Here's how the part is built. I have some questions about the finished solid (model axes, mm). Round coordinates to 2 decimals unless told otherwise and drop trailing zeros. Answer as a JSON object with one key per item and string values.
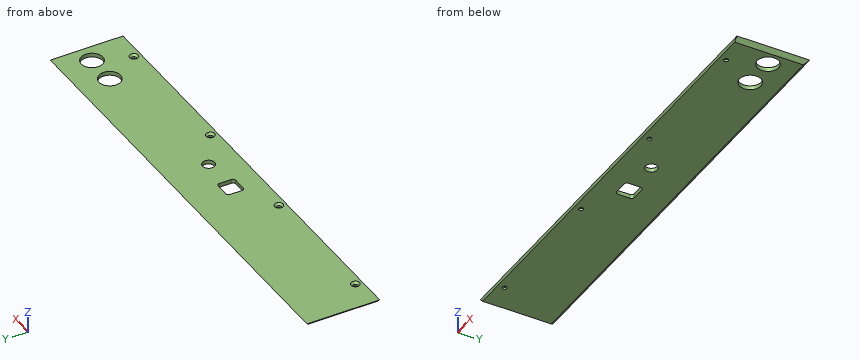
from build123d import *

# Parameters (mm, degrees)
SKETCH1_W                                      = 335.5
SKETCH1_H                                      = 54
BOSS_EXTRUDE1_DEPTH                            = 3
CHAMFER1_SIZE                                  = 3
CSK_FOR_M3_FLAT_HEAD_MACHINE_SCREW1_AT_2_COUNT = 2
CSK_FOR_M3_FLAT_HEAD_MACHINE_SCREW1_AT_2_PITCH = 100
CSK_FOR_M3_FLAT_HEAD_MACHINE_SCREW1_AT_3_COUNT = 2
CSK_FOR_M3_FLAT_HEAD_MACHINE_SCREW1_AT_3_PITCH = 189.5
CSK_FOR_M3_FLAT_HEAD_MACHINE_SCREW1_AT_4_COUNT = 2
CSK_FOR_M3_FLAT_HEAD_MACHINE_SCREW1_AT_4_PITCH = 289.5
SKETCH5_R                                      = 4.5
SKETCH5_R_2                                    = 8
CUT_EXTRUDE1_DEPTH                             = 340.831208102


with BuildPart() as part:
    # Sketch1 → Boss-Extrude1 (new body)
    with BuildSketch(Plane.XY):
        with Locations((167.75, 27)):
            Rectangle(SKETCH1_W, SKETCH1_H)
    extrude(amount=BOSS_EXTRUDE1_DEPTH)

    # Chamfer1
    chamfer1_edges = [part.edges().sort_by_distance(p)[0] for p in [
        (0, 27, 0),
        (167.75, 54, 0),
        (335.5, 27, 0),
    ]]
    chamfer(chamfer1_edges, length=CHAMFER1_SIZE - 0.0001)  # a hair under: the kernel refuses the full size

    # Sketch3 → CSK for M3 Flat Head Machine Screw1 (revolve, cut)
    with BuildSketch(Plane(origin=(23, 5, 3), x_dir=(0, -1, 0), z_dir=(1, 0, 0))):
        Polygon((0, 0), (0, 3), (1.7, 3), (1.7, 1.45), (3.15, 0), align=None)
    csk_for_m3_flat_head_machine_screw1 = revolve(axis=Axis((23, 5, 9.35), (0, 0, -1)), mode=Mode.SUBTRACT)

    # CSK for M3 Flat Head Machine Screw1 at 2: CSK for M3 Flat Head Machine Screw1 ×2
    with Locations(*[(i * CSK_FOR_M3_FLAT_HEAD_MACHINE_SCREW1_AT_2_PITCH, 0, 0) for i in range(1, CSK_FOR_M3_FLAT_HEAD_MACHINE_SCREW1_AT_2_COUNT)]):
        add(csk_for_m3_flat_head_machine_screw1, mode=Mode.SUBTRACT)

    # CSK for M3 Flat Head Machine Screw1 at 3: CSK for M3 Flat Head Machine Screw1 ×2
    with Locations(*[(i * CSK_FOR_M3_FLAT_HEAD_MACHINE_SCREW1_AT_3_PITCH, 0, 0) for i in range(1, CSK_FOR_M3_FLAT_HEAD_MACHINE_SCREW1_AT_3_COUNT)]):
        add(csk_for_m3_flat_head_machine_screw1, mode=Mode.SUBTRACT)

    # CSK for M3 Flat Head Machine Screw1 at 4: CSK for M3 Flat Head Machine Screw1 ×2
    with Locations(*[(i * CSK_FOR_M3_FLAT_HEAD_MACHINE_SCREW1_AT_4_PITCH, 0, 0) for i in range(1, CSK_FOR_M3_FLAT_HEAD_MACHINE_SCREW1_AT_4_COUNT)]):
        add(csk_for_m3_flat_head_machine_screw1, mode=Mode.SUBTRACT)

    # Sketch5 → Cut-Extrude1 (cut, through all)
    with BuildSketch(Plane.XY.offset(3)):
        with Locations((184.9, 22)):
            Circle(SKETCH5_R)
        with Locations((298.7, 30.75)):
            Circle(SKETCH5_R_2)
        with Locations((321.9, 30.75)):
            Circle(SKETCH5_R_2)
        with BuildLine():
            Line((151, 28.5), (161, 28.5))
            ThreePointArc((161, 28.5), (162.414213562, 27.914213562), (163, 26.5))
            Line((163, 26.5), (163, 17.5))
            ThreePointArc((163, 17.5), (162.414213562, 16.085786438), (161, 15.5))
            Line((161, 15.5), (151, 15.5))
            ThreePointArc((151, 15.5), (149.585786438, 16.085786438), (149, 17.5))
            Line((149, 17.5), (149, 26.5))
            ThreePointArc((149, 26.5), (149.585786438, 27.914213562), (151, 28.5))
        make_face()
    extrude(amount=-CUT_EXTRUDE1_DEPTH, mode=Mode.SUBTRACT)


solid = part.part
Item 1: Please list where these lines run through material, in increasing order: probe 1 along X at (y, z) = (6.5, 1.95); probe 2 along X at (y, z) = (18.5, 1.8); probe 3 along X at (y, z) = (5, 1.1). Write a range as from..to.
Resolved:
{"probe 1": "1.05..21.53, 24.47..121.53, 124.47..211.03, 213.97..311.03, 313.97..334.45", "probe 2": "1.2..149, 163..182.07, 187.73..334.3", "probe 3": "1.9..21.3, 24.7..121.3, 124.7..210.8, 214.2..310.8, 314.2..333.6"}
Item 2: I want a section at B-B, the plane y = 35. State how many separate pieces and enclosed holes the cut face has, then the cut area to 3 significant figures.
Resolved:
{"separate pieces": "3", "enclosed holes": "0", "area": "916 mm²"}
Item 3: I'm going to push flat-ended pins straight in: pin 1 Ø1.5 at (y, z) = (23, 2) entering from -X; pin 2 Ø0.9 at (y, z) = (22, 1) entering from +X; pin 3 Ø1.5 at (x, z) = (157.5, 1.5) entering from +Y. Where does each tip first touch, or does it pass through?
Resolved:
{"pin 1": "x = 0.25", "pin 2": "x = 333.95", "pin 3": "y = 53.25"}
